For this review, take the finished solid that the model builds, in its own axes (mm). A direction names the side the tool comes from. Round coordinates to 2 decimals unless told otherwise and drop trailing zeros. Order: outer loops, then holes, each group sorted by start corner. A loop starts at its lowest first (then second) coordinate and runs counter-clockwise, first axis right, second up. Notation, with made-up numbers: (24.5, 58.5) - (31.5, 58.5) arc R36 cw to (31.5, 95.5) - close; hole circle Ø4 at (81.25, 51). An arc over 180 degrees is marked (long way). One line per item, written item: value.
```python
from build123d import *

# Parameters (mm, degrees)
SKETCH_1_R      = 1.6
SKETCH_1_R_2    = 3
EXTRUDE_1_DEPTH = 3


with BuildPart() as part:
    # 草图1 → 凸台-拉伸1 (new body)
    with BuildSketch(Plane(origin=(0, 0, 0), x_dir=(1, 0, 0), z_dir=(0, 1, 0))):
        with BuildLine():
            Line((-97.894892614, -3), (-18.33030278, -3))
            ThreePointArc((-18.33030278, -3), (-15.591689992, -3.816699867), (-13.747727085, -6))
            ThreePointArc((-13.747727085, -6), (0, -15), (13.747727085, -6))
            ThreePointArc((13.747727085, -6), (15.591689992, -3.816699867), (18.33030278, -3))
            Line((18.33030278, -3), (97.894892614, -3))
            ThreePointArc((97.894892614, -3), (99.301864892, -2.421417957), (99.894788276, -1.020429009))
            ThreePointArc((99.894788276, -1.020429009), (0, 99.9), (-99.894788276, -1.020429009))
            ThreePointArc((-99.894788276, -1.020429009), (-99.301864892, -2.421417957), (-97.894892614, -3))
        make_face()
        with Locations(Location((0, 96.9, 0), (0, 0, 270))):
            Circle(SKETCH_1_R, mode=Mode.SUBTRACT)
        with Locations(Location((68.518647097, 68.518647097, 0), (0, 0, 270))):
            Circle(SKETCH_1_R, mode=Mode.SUBTRACT)
        with Locations(Location((96.9, 0, 0), (0, 0, 270))):
            Circle(SKETCH_1_R, mode=Mode.SUBTRACT)
        with Locations(Location((-96.9, 0, 0), (0, 0, 270))):
            Circle(SKETCH_1_R, mode=Mode.SUBTRACT)
        with Locations(Location((-68.518647097, 68.518647097, 0), (0, 0, 270))):
            Circle(SKETCH_1_R, mode=Mode.SUBTRACT)
        with Locations(Location((0, 0, 0), (0, 0, 270))):
            Circle(SKETCH_1_R_2, mode=Mode.SUBTRACT)
        with BuildLine():
            Line((6.081118318, -3.818376618), (7.495331881, -5.232590181))
            ThreePointArc((7.495331881, -5.232590181), (7.495331881, -7.495331881), (5.232590181, -7.495331881))
            Line((5.232590181, -7.495331881), (3.818376618, -6.081118318))
            ThreePointArc((3.818376618, -6.081118318), (3.818376618, -3.818376618), (6.081118318, -3.818376618))
        make_face(mode=Mode.SUBTRACT)
        with BuildLine():
            Line((-3.818376618, -6.081118318), (-5.232590181, -7.495331881))
            ThreePointArc((-5.232590181, -7.495331881), (-7.495331881, -7.495331881), (-7.495331881, -5.232590181))
            Line((-7.495331881, -5.232590181), (-6.081118318, -3.818376618))
            ThreePointArc((-6.081118318, -3.818376618), (-3.818376618, -3.818376618), (-3.818376618, -6.081118318))
        make_face(mode=Mode.SUBTRACT)
        with BuildLine():
            Line((-6.081118318, 3.818376618), (-7.495331881, 5.232590181))
            ThreePointArc((-7.495331881, 5.232590181), (-7.495331881, 7.495331881), (-5.232590181, 7.495331881))
            Line((-5.232590181, 7.495331881), (-3.818376618, 6.081118318))
            ThreePointArc((-3.818376618, 6.081118318), (-3.818376618, 3.818376618), (-6.081118318, 3.818376618))
        make_face(mode=Mode.SUBTRACT)
        with BuildLine():
            Line((3.818376618, 6.081118318), (5.232590181, 7.495331881))
            ThreePointArc((5.232590181, 7.495331881), (7.495331881, 7.495331881), (7.495331881, 5.232590181))
            Line((7.495331881, 5.232590181), (6.081118318, 3.818376618))
            ThreePointArc((6.081118318, 3.818376618), (3.818376618, 3.818376618), (3.818376618, 6.081118318))
        make_face(mode=Mode.SUBTRACT)
        with BuildLine():
            Line((-91.763881784, 3), (-18.33030278, 3))
            ThreePointArc((-18.33030278, 3), (-15.591689992, 3.816699867), (-13.747727085, 6))
            ThreePointArc((-13.747727085, 6), (-10.606601718, 10.606601718), (-6, 13.747727085))
            ThreePointArc((-6, 13.747727085), (-3.816699867, 15.591689992), (-3, 18.33030278))
            Line((-3, 18.33030278), (-3, 91.763881784))
            ThreePointArc((-3, 91.763881784), (-3.624795989, 93.216057368), (-5.108813928, 93.760919472))
            ThreePointArc((-5.108813928, 93.760919472), (-66.397326753, 66.397326753), (-93.760919472, 5.108813928))
            ThreePointArc((-93.760919472, 5.108813928), (-93.216057368, 3.624795989), (-91.763881784, 3))
        make_face(mode=Mode.SUBTRACT)
        with BuildLine():
            Line((3, 18.33030278), (3, 91.763881784))
            ThreePointArc((3, 91.763881784), (3.624795989, 93.216057368), (5.108813928, 93.760919472))
            ThreePointArc((5.108813928, 93.760919472), (66.397326753, 66.397326753), (93.760919472, 5.108813928))
            ThreePointArc((93.760919472, 5.108813928), (93.216057368, 3.624795989), (91.763881784, 3))
            Line((91.763881784, 3), (18.33030278, 3))
            ThreePointArc((18.33030278, 3), (15.591689992, 3.816699867), (13.747727085, 6))
            ThreePointArc((13.747727085, 6), (10.606601718, 10.606601718), (6, 13.747727085))
            ThreePointArc((6, 13.747727085), (3.816699867, 15.591689992), (3, 18.33030278))
        make_face(mode=Mode.SUBTRACT)
    extrude(amount=EXTRUDE_1_DEPTH)


solid = part.part
```
Item 1: Take a section at D-D (y = 0.8). Count the separate pieces of the cut face and the enclosed holes in it, plus the area to 3 significant figures.
Returned:
separate pieces: 1
enclosed holes: 12
area: 3,880 mm^2
Item 2: Take a section at B-B (z = -30). Write out the cut boundary in (x, y).
Returned:
outline: (-95.29, 0) - (-88.98, 0) - (-88.98, 3) - (-95.29, 3) - close; (-3, 0) - (3, 0) - (3, 3) - (-3, 3) - close; (88.98, 0) - (95.29, 0) - (95.29, 3) - (88.98, 3) - close
Item 3: For P1, Ø12, axis at x = 78.5, z = -26.5, coming from the -Y side; P2, Ø1.5, axis at y = 1, z = -45, coming from the -X side; P3, Ø0.9, axis at x = 47, y = 1.5, coming from the +Z side; P4, Ø0.9, axis at x = 37.5, y = 1, coming from the -Z side, all flat-tipped, find the tip position at first contact; note any pin that passes through.
Returned:
P1: through
P2: x = -89.57
P3: z = 3
P4: z = -92.78
Item 4: Take a section at C-C (z = -62). Write out the cut boundary in (x, y), plus the area to 3 significant figures.
Returned:
outline: (-78.33, 0) - (-70.52, 0) - (-70.52, 3) - (-78.33, 3) - close; (-3, 0) - (3, 0) - (3, 3) - (-3, 3) - close; (70.52, 0) - (78.33, 0) - (78.33, 3) - (70.52, 3) - close
area: 64.9 mm^2
Item 5: Machinability: for faces 1 (the cylindrical face through (-65.714, 1.479, -67.073)), 2 (the flat face through (0, 3, -34)), which of the approach directions +Z, -Z, +X, -X, +Y, -Y give a long, thin tool a straight path to every point of the face, cutting with its end or side? Answer none if there is none.
Returned:
face 1: +Y, -Y
face 2: +Z, -Z, +X, -X, +Y
Item 6: Take a section at A-A (x = 29). Write out the cut boundary in (y, z), plus the area to 3 significant figures.
Returned:
outline: (0, -95.6) - (3, -95.6) - (3, -89.31) - (0, -89.31) - close; (0, -3) - (3, -3) - (3, 3) - (0, 3) - close
area: 36.9 mm^2
Item 7: Wall thickness on line 1 (X direction, y = 1.05, z = 0); line 2 (X direction, y = 1.55, z = -64); line 3 (X direction, y = 1.4, z = -27): over which ranges is each line inside the solid? List them lowest first.
Returned:
line 1: -99.9 to -98.5, -95.3 to -3, 3 to 95.3, 98.5 to 99.9
line 2: -76.71 to -68.71, -3 to 3, 68.71 to 76.71
line 3: -96.18 to -89.93, -3 to 3, 89.93 to 96.18
